Geometry: see drawing. Coordinates: mm, zero at the bounding-box minimum. Coordinates: 2 decimals unless noted, no trailing zeros. Order: outer loops, then holes, each group sorted by start corner. A loop starts at its lowest first (then second) coordinate and runs counter-clockwise, first axis right, second up.
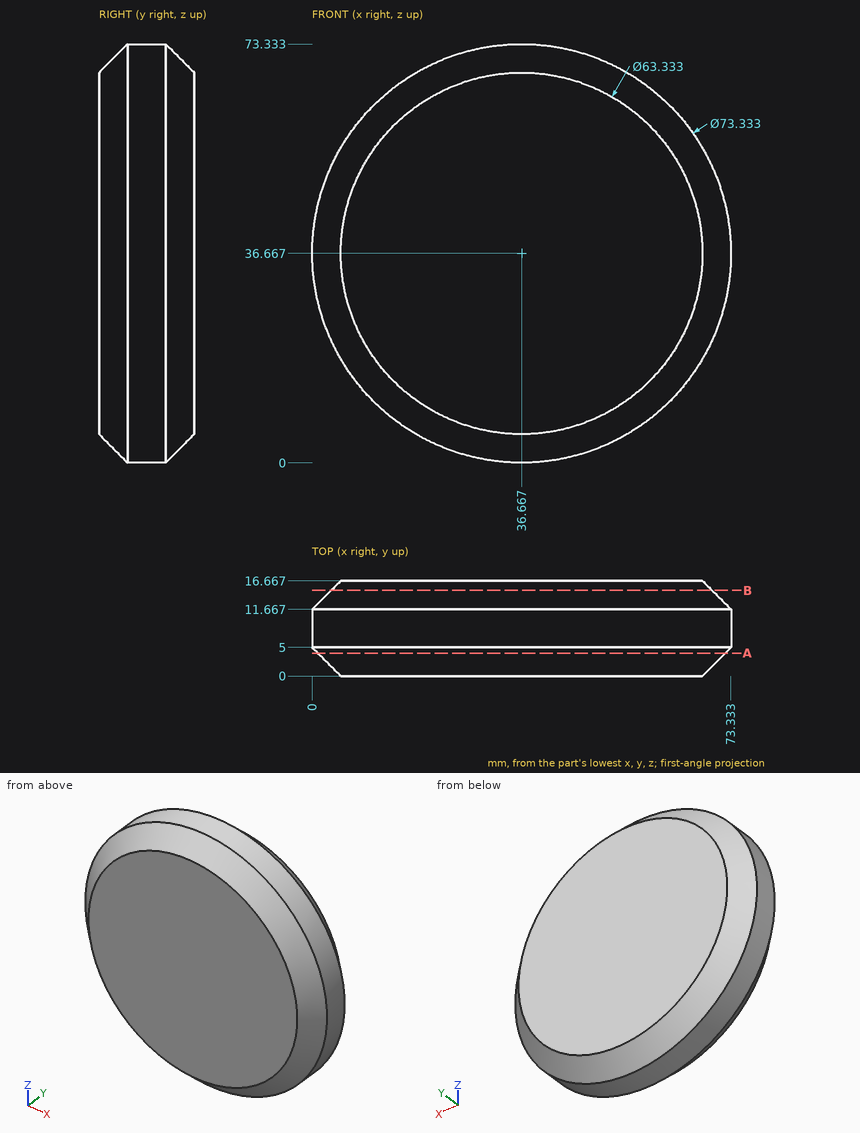
Item 1: Pin query (flat end, axial travel): pin 1 Ø8 at (y, z) = (3.5, 60) entering from +X; pin 2 Ø6 at (x, z) = (51.5, 61.5) entering from -Y; pin 3 Ø2 at (x, y) = (9.5, 8.5) entering from +Z; pin 4 Ø1 at (x, y) = (37.5, 12) entering from +Z. Return the tip coordinate at first contact, or that it passes through.
Response values:
pin 1: stops at x = 67.64
pin 2: stops at y = 0
pin 3: stops at z = 62.35
pin 4: stops at z = 73.33
Item 2: Cut plane A-A on y = 4. Return loops of the section in (x, z), then the cut area to 3 significant figures.
Response values:
outline: circle Ø71.33 at (36.67, 36.67)
area: 4,000 mm2
Item 3: Cut plane B-B on y = 15. Return loops of the section in (x, z), then the cut area to 3 significant figures.
Response values:
outline: circle Ø66.67 at (36.67, 36.67)
area: 3,490 mm2
Item 4: Ray query, probe 1 along Z at (x, y) = (51, 12.5) (1 decimal); probe 2 along X at (y, z) = (4.5, 37); probe 3 along Y at (x, z) = (50, 68) (1 decimal). Return the intervals inside material, ascending.
Response values:
probe 1: z = 3.8 to 69.5
probe 2: x = 0.5 to 72.83
probe 3: y = 2.4 to 14.3
